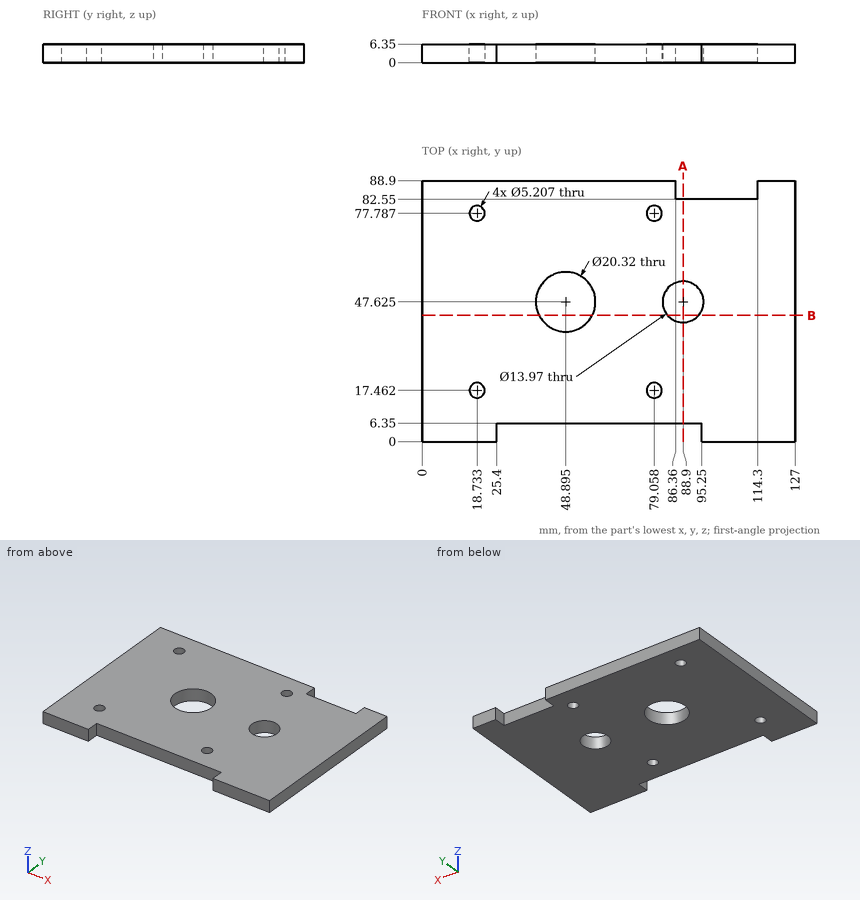
The figure shows three views and two pictorial views of one solid part (mm, origin at its lowest corner). Answer the questions. Give positions to 0.01 mm unless a question says otherwise; leave off trailing zeros. Loops run counter-clockwise (first coordinate to the right, second up) from the corner with the lowest first, then second, coordinate; pieces in that order, holes last. Notation, with made-up numbers: (-11, 87) -> (47, 87) arc R29 ccw to (47, 117) -> close; hole circle Ø4 at (48, 49). An arc over 180 degrees is marked (long way). Use a Markdown table: item, result. Add a question column.
1. Flat-ended cylindrical pins translate along their axes: pin 1 Ø1.9 at (x, z) = (77, 4.5) entering from -Y; pin 2 Ø3 at (y, z) = (86, 3.5) entering from -X. Find the tip coordinate at first contact, or state that the pin passes through.
2. Section A-A on x = 88.9 is taken. Determine the outline of the cut face in (y, z), and give its area (3 significant figures).
3. Find the intervals of material crossed by probe 1 along X at (y, z) = (77.5, 1.5) (1 decimal); probe 2 along X at (y, z) = (17.5, 6.25) (1 decimal); probe 3 along X at (y, z) = (85, 5.5), in increasing order.
4. Section B-B on y = 43 is taken. State how many separate pieces and enclosed holes the cut face has, and give its area (3 significant figures).
Results below:
| question | item | result |
|---|---|---|
| 1 | pin 1 | stops at y = 6.35 |
| 1 | pin 2 | stops at x = 0 |
| 2 | outline | (6.35, 0) -> (40.64, 0) -> (40.64, 6.35) -> (6.35, 6.35) -> close; (54.61, 0) -> (82.55, 0) -> (82.55, 6.35) -> (54.61, 6.35) -> close |
| 2 | area | 395 mm^2 |
| 3 | probe 1 | x = 0 to 16.1, 21.3 to 76.5, 81.6 to 127 |
| 3 | probe 2 | x = 0 to 16.1, 21.3 to 76.5, 81.7 to 127 |
| 3 | probe 3 | x = 0 to 86.36, 114.3 to 127 |
| 4 | separate pieces | 3 |
| 4 | enclosed holes | 0 |
| 4 | area | 625 mm^2 |
